Part model, mm, in its own coordinate system. A direction names the side the tool comes from. Round coordinates to 2 decimals unless told otherwise and drop trailing zeros. Write each loop counter-clockwise with the first axis right and the second up, starting at its lowest first coordinate (ties: lowest second). Pieces come first, ordered by that corner, then holes. Notation, with made-up numbers: M 61,25.25 L 110,25.25 A6 cw 110,35.25 Z; hole C -37.75,35 d1. An arc over 180 degrees is marked long. One line per question, with ' | ' between items. Start each with the question number.
1) Mould opens along X. For faces 4 (the face through (-3.445, 12.325, -93.937)), 5 (the face through (-0.3, 24.5, 35)), 6 (the face through (1, 25, -5)) say: pulls with the +X half, pulls with the -X half, needs draft (parallel to the pull), parting line crosses it, or undercut.
2) Tool access for faces 1 (the face through (22.843, 22.375, 32.566)), 2 (the face through (22, 18, 35)), 3 (the face through (21.81, 19.57, 34.23)): list every direction of +Z, -Z, +X, -X, +Y, -Y with a clear straight run to the whole face (end or side of a thin tool).
3) Saw through at C-C (x = 0). List the corners of the cut face in (y, z).
4) Saw through at D-D (y = 8.75). List the corners of the cut face in (x, z), plus the area to 3 significant figures.
5) Saw through at B-B (z = 45). List the corners of the cut face in (x, y).
6) Wall check: probe 1 along X at (y, z) = (19, 0); probe 2 along Y at (x, z) = (51, 37.5); probe 3 along X at (y, z) = (21.75, -3). Give the ranges that are in metal, low to high. Write a range as [from, to].
7) Saw through at A-A (z = 0). List the corners of the cut face in (x, y), plus the area to 3 significant figures.
8) Drop flat-ended pins along their axis: pin 1 Ø8 at (y, z) = (4.5, 6) entering from -X; pin 2 Ø3.5 at (x, z) = (31.5, -16) entering from -Y; pin 3 Ø6 at (y, z) = (8, -33.5) entering from -X. Give the stop position or say it passes through.
Autodesk Inventor part; units mm, degrees
ref_plane "YZ Plane" through (0, 0, 0) normal (1, 0, 0) x (0, 1, 0)
ref_plane "XZ Plane" through (0, 0, 0) normal (0, 1, 0) x (-1, 0, 0)
ref_plane "XY Plane" through (0, 0, 0) normal (0, 0, 1) x (1, 0, 0)
sketch "Sketch1" plane through (0, 0, 0) normal (0, 1, 0) x (-1, 0, 0)
  circle A0 centre (0, 0) radius 94
  dimension "d0" = 188
extrude "Extrusion1" add sketch "Sketch1" along normal blind 25
sketch "Sketch2" plane through (0, 0, 0) normal (0, -1, 0) x (1, 0, 0)
  point P0 (0, 0)
  point P1 (0, 0)
hole "Hole1" at (0, 0, 0) direction (0, 1, 0) diameter 186 depth 24
sketch "Sketch11" plane through (0, 25, 0) normal (0, 1, 0) x (1, 0, 0)
  circle A0 centre (0, 0) radius 94.1047
  circle A1 centre (0, 0) radius 35
  line L0 (35, 0) -> (94.1047, 0)
  line L1 (17.5, 30.3109) -> (47.0523, 81.4971)
  line L2 (-17.5, 30.3109) -> (-47.0523, 81.4971)
  line L3 (-35, 0) -> (-94.1047, 0)
  line L4 (-17.5, -30.3109) -> (-47.0523, -81.4971)
  line L5 (17.5, -30.3109) -> (47.0523, -81.4971)
  dimension "d46" = 70
  dimension "d49" = 360
extrude "Extrusion4" cut sketch "Sketch11" against normal blind 30 contours A0 L4 A1 L5
sketch "Sketch5" plane through (0, 24, 0) normal (0, -1, 0) x (1, 0, 0)
  circle A0 centre (0.0185, 0.5394) radius 32.5
  circle A1 centre (0.0185, 0.5394) radius 91
  line L0 (0.0185, -31.9606) -> (0.0185, -90.4606)
  line L1 (-28.1273, -15.7106) -> (-78.7898, -44.9606)
  line L2 (-28.1273, 16.7894) -> (-78.7898, 46.0394)
  line L3 (0.0185, 33.0394) -> (0.0185, 91.5394)
  line L4 (28.1643, 16.7894) -> (78.8268, 46.0394)
  line L5 (27.2527, -15.1843) -> (78.8268, -44.9606)
  line L6 (30.5108, -13.5333) -> (27.5108, -18.7294)
  line L7 (27.5108, -18.7294) -> (31.8409, -21.2294)
  line L8 (31.8409, -21.2294) -> (34.8409, -16.0333)
  line L9 (34.8409, -16.0333) -> (30.5108, -13.5333)
  line L10 (-2.9302, -37.8595) -> (3.0698, -37.8595)
  line L11 (3.0698, -32.8595) -> (-2.9302, -32.8595)
  line L12 (-2.9302, -32.8595) -> (-2.9302, -37.8595)
  line L13 (3.0698, -37.8595) -> (3.0698, -32.8595)
  point P0 (0, 0)
  point P1 (24.0416, -20.6125)
  point P2 (3.0698, -35.3595)
  dimension "d23" = 65
  dimension "d30" = 360
  dimension "d38" = 6
  dimension "d39" = 5
  dimension "d40" = 6
  dimension "d41" = 5
extrude "Extrusion3" add sketch "Sketch5" along normal blind 0.1 contours L6 L9 L8 L5 | L5 L8 L7 L6 | L11 L13 L10 L0 | L0 L10 L12 L11
sketch "Sketch12" plane through (-47, 0, 81.4064) normal (0.8660254, 0, 0.5) x (0.5, 0, -0.8660254)
  point P0 (94, 0)
sketch "Sketch13" plane through (-47, 0, 81.4064) normal (0.8660254, 0, 0.5) x (0.5, 0, -0.8660254)
  line L0 (59, 24) -> (1, 24)
  line L1 (50, 24) -> (56, 24)
  line L2 (56, 24) -> (56, 18)
  line L3 (56, 18) -> (50, 18)
  line L4 (50, 18) -> (50, 24)
  line L5 (59, 25) -> (59, 24)
  point P0 (94, 0)
  dimension "d53" = 6
  dimension "d54" = 6
  dimension "d55" = 3
extrude "Extrusion5" add sketch "Sketch13" against normal blind 3.5
sketch "Sketch14" plane through (-47, 0, 81.4064) normal (0.8660254, 0, 0.5) x (0.5, 0, -0.8660254)
  circle A0 centre (53, 21) radius 1.5
  line L0 (50, 24) -> (50, 18)
  line L1 (50, 18) -> (56, 18)
  point P0 (94, 0)
  dimension "d58" = 3
  dimension "d59" = 3
  dimension "d60" = 3
hole "Hole2" at (-20.5, 21, 35.507) direction (-0.8660254, 0, -0.5) diameter 3 depth 29
sketch "Sketch15" plane through (47, 0, 81.4064) normal (-0.8660254, 0, 0.5) x (0.5, 0, 0.8660254)
  line L0 (-56, 24) -> (-50, 24)
  line L1 (-50, 24) -> (-50, 18)
  line L2 (-50, 18) -> (-56, 18)
  line L3 (-56, 18) -> (-56, 24)
  line L4 (-59, 25) -> (-59, 24)
  line L5 (-1, 24) -> (-59, 24)
  point P0 (-94, 0)
  dimension "d68" = 6
  dimension "d69" = 6
  dimension "d70" = 3
  dimension "d71" = 0
extrude "Extrusion6" add sketch "Sketch15" against normal blind 3.5
sketch "Sketch16" plane through (47, 0, 81.4064) normal (-0.8660254, 0, 0.5) x (0.5, 0, 0.8660254)
  circle A0 centre (-53, 21) radius 1.5
  line L0 (-56, 24) -> (-56, 18)
  line L1 (-50, 24) -> (-56, 24)
  point P0 (-94, 0)
  dimension "d74" = 3
  dimension "d75" = 3
  dimension "d76" = 3
hole "Hole3" at (20.5, 21, 35.507) direction (0.8660254, 0, -0.5) diameter 3 depth 29
properties part number "Cover"
Answer key:
1) face 4: parting line crosses it | face 5: undercut | face 6: needs draft
2) face 1: -Y | face 2: +Z, -Y | face 3: none
3) outline: M 0,-94 L 25,-94 L 25,35 L 24,35 L 24,-32.86 L 23.9,-32.86 L 23.9,-37.86 L 24,-37.86 L 24,-93 L 0,-93 Z
4) outline: M -47,81.41 A94 ccw long 47,81.41 L 46.5,80.54 A93 cw long -46.5,80.54 Z | area: 490 mm2
5) outline: M -82.53,0 L -81.39,0 L -81.39,24 L -25.98,24 L -25.98,25 L -82.53,25 Z; M 25.98,24 L 81.39,24 L 81.39,0 L 82.53,0 L 82.53,25 L 25.98,25 Z
6) probe 1: x = [-94, -93], [93, 94] | probe 2: y = [24, 25] | probe 3: x = [-93.95, -92.95], [92.95, 93.95]
7) outline: M -94,0 L -93,0 L -93,24 L 93,24 L 93,0 L 94,0 L 94,25 L -94,25 Z | area: 236 mm2
8) pin 1: stops at x = -93.98 | pin 2: stops at y = 23.9 | pin 3: stops at x = -88.91
